Autodesk Inventor part; units mm, degrees
ref_plane "YZ Plane" through (0, 0, 0) normal (1, 0, 0) x (0, 1, 0)
ref_plane "XZ Plane" through (0, 0, 0) normal (0, 1, 0) x (-1, 0, 0)
ref_plane "XY Plane" through (0, 0, 0) normal (0, 0, 1) x (1, 0, 0)
sketch "Sketch1" plane through (0, 0, 0) normal (0, 0, 1) x (1, 0, 0)
  line L0 (0, 0) -> (0, 4)
  line L1 (0, 4) -> (15, 4)
  line L2 (15, 4) -> (15, 8)
  line L3 (15, 8) -> (-3, 8)
  line L4 (-3, 8) -> (-3, 0)
  line L5 (0, 0) -> (0, -4)
  line L6 (0, -4) -> (15, -4)
  line L7 (15, -4) -> (15, -8)
  line L8 (15, -8) -> (-3, -8)
  line L9 (-3, -8) -> (-3, 0)
  point P0 (0, 2)
  dimension "d4" = 3
  dimension "d5" = 4
  dimension "d17" = 15
extrude "Extrusion1" add sketch "Sketch1" along normal blind 8
sketch "Sketch2" plane through (-3, 8, 0) normal (0, 1, 0) x (1, 0, 0)
  circle A0 centre (14, -4) radius 2
  line L0 (18, 0) -> (18, -8)
  point P0 (3, 0)
  point P1 (18, -4)
  dimension "d8" = 4
  dimension "d9" = 4
extrude "Extrusion2" cut sketch "Sketch2" against normal through all
fillet "Fillet1" radius 4 4 edges at (15, 6, 8) (15, 6, 0) (15, -6, 8) (15, -6, 0)
sketch "Sketch3" plane through (0, -4, 0) normal (1, 0, 0) x (0, 0, -1)
  circle A0 centre (-4, 4) radius 2.5
  line L0 (0, 0) -> (0, 8)
  point P0 (0, 4)
  point P1 (0, 4)
  dimension "d13" = 5
  dimension "d14" = 4
extrude "Extrusion3" cut sketch "Sketch3" against normal blind 10
properties part number "actuator mount 2"
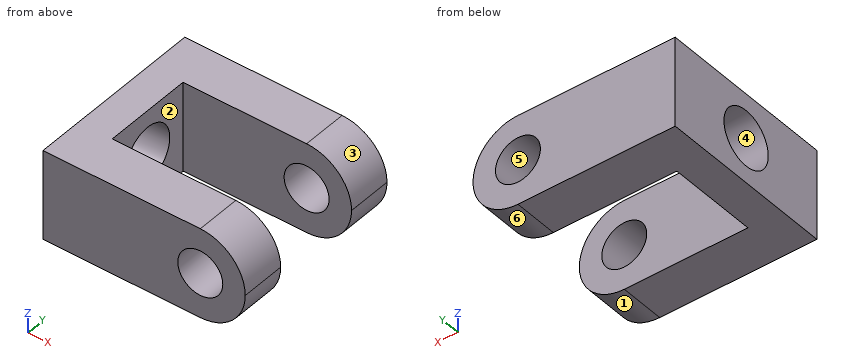
Model file for the job. Use its own axes, mm. Face numbers are marked on the shaded views. A direction names the side the tool comes from. Give positions to 0.01 mm unless a question says otherwise; leave off trailing zeros. Order: outer loops, then holes, each group sorted by start corner. A loop starts at its lowest first (then second) coordinate and runs counter-clockwise, first axis right, second up. Notation, with made-up numbers: M 41,40.5 L 75,40.5 A23 ccw 75,48.5 Z; hole C 51,70 d1. An arc over 180 degrees is marked long. Put each result on its own line as item: value. Start each with the question number.
(1) Pull direction Z, two halves, no side cores. Call the marked faces 3, 4, 5 and 6: released by +Z, released by -Z, zero draft, split by the parting line, or undercut.
(2) Drill centre lines: L1, parallel to Y at x = 9.25, z = 2; L2, parallel to Z at x = 11, y = 5.6; L3, parallel to X at y = 6.95, z = 4. Where is each one in solid material? Low to high. Write a range as [from, to].
(3) Pin check, flat tip, straight feed: pin 1 Ø1.5 at (y, z) = (-3, 6) entering from +X. Stop position of the tip, or through.
(4) Tool access for the marked faces 1 and 2: list every direction of +Z, -Z, +X, -X, +Y, -Y with a clear straight run to the whole face (end or side of a thin tool).
(5) Band-saw the part on A-A on y = 0. Give the cut face in (x, z), then the cut area to 3 significant figures.
(6) Band-saw the part on B-B on x = 7.5. Give the cut face in (y, z), then the cut area to 3 significant figures.
(7) Band-saw the part on D-D on z = 4.5. Give the cut face in (x, y), then the cut area to 3 significant figures.
Results below:
1. face 3: released by +Z
1. face 4: undercut
1. face 5: undercut
1. face 6: released by -Z
2. L1: y = [-8, -4], [4, 8]
2. L2: z = [0, 2], [6, 8]
2. L3: x = [-3, 9], [13, 15]
3. pin 1: stops at x = 0
4. face 1: -Z, +X, +Y, -Y
4. face 2: +Z, -Z, +X
5. outline: M -3,0 L 0,0 L 0,1.5 L -3,1.5 Z; M -3,6.5 L 0,6.5 L 0,8 L -3,8 Z
5. area: 9.00 mm2
6. outline: M -8,0 L -4,0 L -4,8 L -8,8 Z; M 4,0 L 8,0 L 8,8 L 4,8 Z
6. area: 64.0 mm2
7. outline: M -3,-8 L 9.06,-8 L 9.06,-4 L 0,-4 L 0,-2.45 L -3,-2.45 Z; M -3,2.45 L 0,2.45 L 0,4 L 9.06,4 L 9.06,8 L -3,8 Z; M 12.94,-8 L 14.97,-8 L 14.97,-4 L 12.94,-4 Z; M 12.94,4 L 14.97,4 L 14.97,8 L 12.94,8 Z
7. area: 122 mm2
